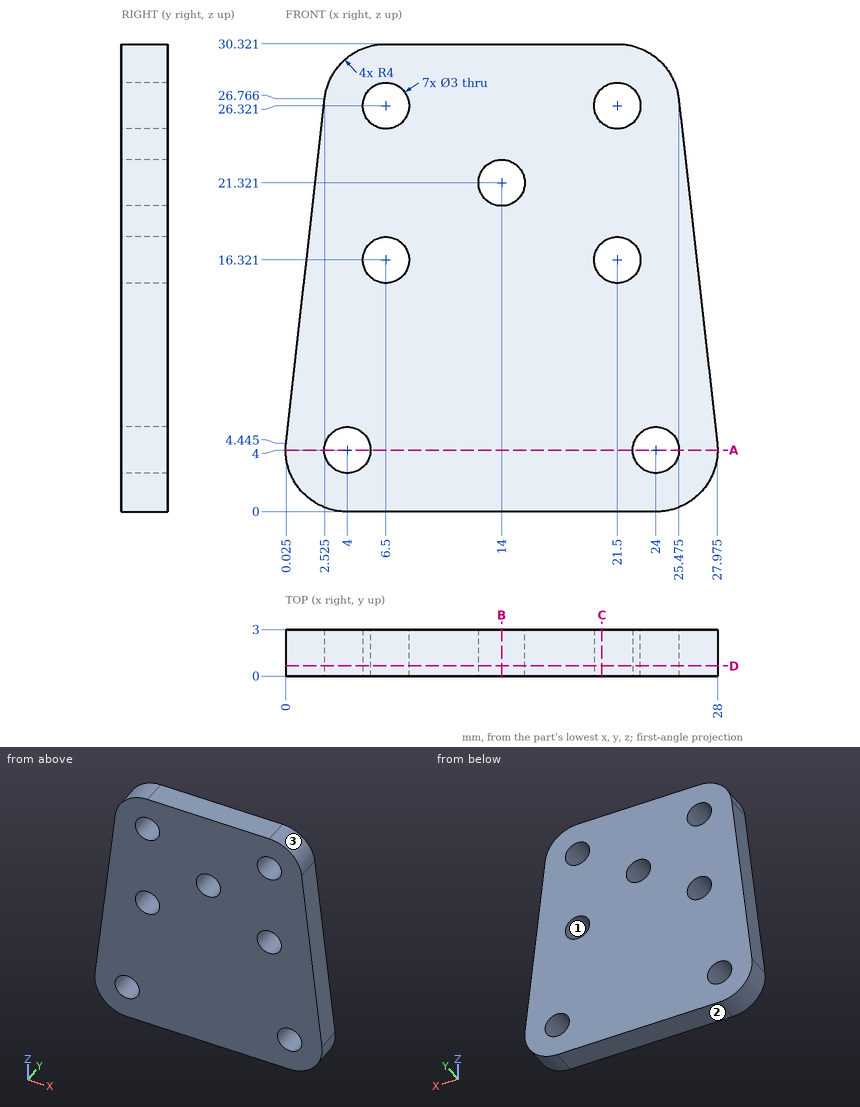
Here's the drawing with two shaded views (mm, measured from the low corner). I have some questions. Give positions to 0.01 mm unless a question says otherwise; leave off trailing zeros. Write each loop counter-clockwise with the first axis right and the second up, starting at its lowest first coordinate (ties: lowest second). Pieces come first, ordered by that corner, then holes. Notation, with made-up numbers: (-20.5, 57) -> (2.5, 57) arc R28 ccw to (2.5, 84) -> close; hole circle Ø6 at (-31.75, 13.5). An arc over 180 degrees is marked (long way). Use one line per item in the form item = value. Start each with the question number.
1. Thinking about a two-plate mould opening in Z: for the marked faces 1, 2 and 3, which applies, +Z half, -Z half, draft (parallel to the pull), parting line (faces both ways), or undercut?
2. If I drill on L1, parallel to Z at x = 21.5, y = 1.15; L2, parallel to X at y = 2.4, z = 4; L3, parallel to Z at x = 7.25, y = 1.9, over which ranges is the centre line in solid material (lowest first)?
3. Imagine slicing it at A-A on z = 4. List the corners of the cut face in (x, y) for me.
4. Imagine slicing it at D-D on y = 0.65. List the corners of the cut face in (x, z) for me (1 decimal), plus the area to 3 significant figures.
5. Imagine slicing it at C-C on x = 20.5. List the corners of the cut face in (y, z) for me.
6. Will these pins go through, and if not, where does the flat tip stop? pin 1 Ø1 at (y, z) = (2.5, 9) entering from +X; pin 2 Ø1.5 at (y, z) = (2.5, 13.5) entering from +X (1 decimal).
7. Imagine slicing it at B-B on x = 14. List the corners of the cut face in (y, z) for me.
Entries:
q1.face_1 = undercut
q1.face_2 = -Z half
q1.face_3 = +Z half
q2.L1 = 0 to 14.82, 17.82 to 24.82, 27.82 to 30.32
q2.L2 = 0 to 2.5, 5.5 to 22.5, 25.5 to 28
q2.L3 = 0 to 15.02, 17.62 to 25.02, 27.62 to 30.32
q3.outline = (0, 0) -> (2.5, 0) -> (2.5, 3) -> (0, 3) -> close; (5.5, 0) -> (22.5, 0) -> (22.5, 3) -> (5.5, 3) -> close; (25.5, 0) -> (28, 0) -> (28, 3) -> (25.5, 3) -> close
q4.outline = (0, 4.4) arc R4 ccw to (4, 0) -> (24, 0) arc R4 ccw to (28, 4.4) -> (25.5, 26.8) arc R4 ccw to (21.5, 30.3) -> (6.5, 30.3) arc R4 ccw to (2.5, 26.8) -> close; hole circle Ø3 at (4, 4); hole circle Ø3 at (6.5, 16.3); hole circle Ø3 at (6.5, 26.3); hole circle Ø3 at (14, 21.3); hole circle Ø3 at (21.5, 16.3); hole circle Ø3 at (21.5, 26.3); hole circle Ø3 at (24, 4)
q4.area = 711 mm²
q5.outline = (0, 0) -> (3, 0) -> (3, 15.2) -> (0, 15.2) -> close; (0, 17.44) -> (3, 17.44) -> (3, 25.2) -> (0, 25.2) -> close; (0, 27.44) -> (3, 27.44) -> (3, 30.32) -> (0, 30.32) -> close
q6.pin_1 = 27.52
q6.pin_2 = 27
q7.outline = (0, 0) -> (3, 0) -> (3, 19.82) -> (0, 19.82) -> close; (0, 22.82) -> (3, 22.82) -> (3, 30.32) -> (0, 30.32) -> close
